```python
from build123d import *

# Parameters (mm, degrees)
BOSS_EXTRUDE1_DEPTH = 6.604
CUT_EXTRUDE1_DEPTH  = 7.604
BOSS_EXTRUDE2_DEPTH = 6.604


with BuildPart() as part:
    # Sketch1 → Boss-Extrude1 (new body)
    with BuildSketch(Plane(origin=(0, 0, 0), x_dir=(0, 0, -1), z_dir=(1, 0, 0))):
        Polygon((0, 0), (-34.925, 60.491874454), (36.917048969, 132.333923423), (54.877561211, 114.373411181), align=None)
    extrude(amount=-BOSS_EXTRUDE1_DEPTH)

    # Sketch2 → Cut-Extrude1 (cut, through all)
    with BuildSketch(Plane(origin=(0, 0, 0), x_dir=(0, 0, -1), z_dir=(1, 0, 0))):
        Polygon((31.654618882, 118.091237215), (27.164490821, 122.581365275), (24.218966813, 119.635841268), (28.709094874, 115.145713207), (27.092648772, 113.529267105), (31.295408637, 109.326507241), (32.911854739, 110.942953343), (33.917643424, 109.937164657), (36.863167432, 112.882688665), (35.857378746, 113.88847735), (37.473824848, 115.504923452), (33.271064983, 119.707683317), align=None)
        Polygon((-13.246661724, 73.18995661), (-17.736789784, 77.68008467), (-20.682313792, 74.734560662), (-16.192185731, 70.244432602), (-17.808631833, 68.6279865), (-13.605871969, 64.425226635), (-11.989425867, 66.041672737), (-10.983637181, 65.035884052), (-8.038113174, 67.981408059), (-9.043901859, 68.987196745), (-7.427455757, 70.603642847), (-11.630215622, 74.806402711), align=None)
        Polygon((-17.382330096, 54.69427888), (-18.525330096, 56.674012953), (-23.672638686, 53.702212953), (-22.529638686, 51.72247888), (-28.0289, 48.54747888), (-25.9461, 44.939963458), (-20.446838686, 48.114963458), (-19.303838686, 46.135229385), (-14.156530096, 49.107029385), (-15.299530096, 51.086763458), (-14.067695562, 51.797963458), (-16.150495562, 55.40547888), align=None)
        Polygon((-2.650330096, 29.177706383), (-7.797638686, 26.205906383), (-6.654638686, 24.22617231), (-12.1539, 21.05117231), (-10.0711, 17.443656888), (-4.571838686, 20.618656888), (-3.428838686, 18.638922815), (1.718469904, 21.610722815), (0.575469904, 23.590456888), (1.807304438, 24.301656888), (-0.275495562, 27.90917231), (-1.507330096, 27.19797231), align=None)
    extrude(amount=-CUT_EXTRUDE1_DEPTH, mode=Mode.SUBTRACT)

    # Sketch3 → Boss-Extrude2 (add)
    with BuildSketch(Plane(origin=(0, 0, 0), x_dir=(0, 0, -1), z_dir=(1, 0, 0))):
        Polygon((30.002251755, 134.758592576), (34.671984938, 130.088859393), (30.181856878, 125.598731332), (25.512123695, 130.268464515), align=None)
        Polygon((21.201600757, 116.618475211), (16.531867574, 121.288208394), (12.041739513, 116.798080333), (16.711472696, 112.12834715), align=None)
        Polygon((-14.719423728, 80.697450727), (-19.389156911, 85.36718391), (-14.89902885, 89.85731197), (-10.229295667, 85.187578787), align=None)
        Polygon((-28.369413032, 76.386927789), (-32.859541092, 71.896799728), (-28.189807909, 67.227066545), (-23.699679849, 71.717194606), align=None)
        Polygon((-39.056731767, 54.440243797), (-33.3375, 57.742243797), (-30.1625, 52.242982483), (-35.881731767, 48.940982483), align=None)
        Polygon((-23.8125, 41.244459855), (-29.531731767, 37.942459855), (-26.356731767, 32.443198541), (-20.6375, 35.745198541), align=None)
        Polygon((-23.181731767, 26.943937227), (-17.4625, 30.245937227), (-14.2875, 24.746675913), (-20.006731767, 21.444675913), align=None)
        Polygon((-13.656731767, 10.446153285), (-10.481731767, 4.946891971), (-4.7625, 8.248891971), (-7.9375, 13.748153285), align=None)
    extrude(amount=-BOSS_EXTRUDE2_DEPTH)


solid = part.part
```
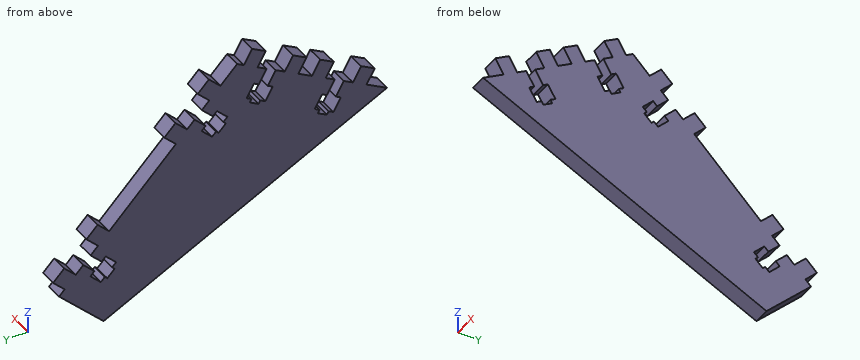
The model under review builds one solid part; all positions refer to its coordinate system, in mm. Give positions to 0.01 mm unless a question says otherwise; leave off trailing zeros. Write each loop counter-clockwise with the first axis right and the second up, starting at its lowest first coordinate (ties: lowest second). Pieces come first, ordered by that corner, then holes.
(1) To check wall thickness, follow L1, parallel to Y at x = -5, z = 17; L2, parallel to Z at x = -5.5, y = 119; L3, parallel to Z at x = -5, y = 73. State the ranges of each line that lie inside material, in increasing order.
(2) Consider section B-B, the plane y = 98.5. Give the boundary of the cut face in (x, z), and give its area (3 significant figures).
(3) For P1, Ø10, axis at y = 63, z = 5, coming from the +X side; P2, Ø1.5, axis at x = -6, z = -23, coming from the +Y side, all flat-tipped, find the tip position at first contact; note any pin that passes through.
(4) Consider section A-A, the plane z = -14. Give the boundary of the cut face in (x, y), and give its area (3 significant figures).
(5) Consider section C-C, the plane z = -44. Give the boundary of the cut face in (x, y), and give its area (3 significant figures).
Returned:
1. L1: y = 23.18 to 47.47, 54.92 to 67.82, 69.44 to 71.05, 76.94 to 78.42, 82.98 to 87.76
1. L2: z = -50.25 to -33.98, -32.56 to -30.75, -24.85 to -23.58, -18.82 to -14.24
1. L3: z = -35.03 to 9.82, 18.95 to 22.42, 24.98 to 31.76
2. outline: (-6.6, -47.26) - (0, -47.26) - (0, -3.08) - (-6.6, -3.08) - close
2. area: 292 mm2
3. P1: stops at x = 0
3. P2: stops at y = 119.17
4. outline: (-6.6, 29.18) - (0, 29.18) - (0, 109.42) - (-6.6, 109.42) - close; (-6.6, 114.84) - (0, 114.84) - (0, 118.76) - (-6.6, 118.76) - close
4. area: 556 mm2
5. outline: (-6.6, 91.7) - (0, 91.7) - (0, 125.25) - (-6.6, 125.25) - close
5. area: 222 mm2
